Drawing for the job (mm, zero at the part's lowest x, y, z). Round coordinates to 2 decimals unless told otherwise and drop trailing zeros. Order: outer loops, then holes, each group sorted by start corner. A loop starts at its lowest first (then second) coordinate and runs counter-clockwise, first axis right, second up. Notation, with made-up numbers: (13, -13) -> (46, -13) arc R21 cw to (46, -9) -> close; hole circle Ø2 at (-18.5, 77). An arc over 180 degrees is marked (long way). Use CSV: the item, a comma, the result in double quotes.
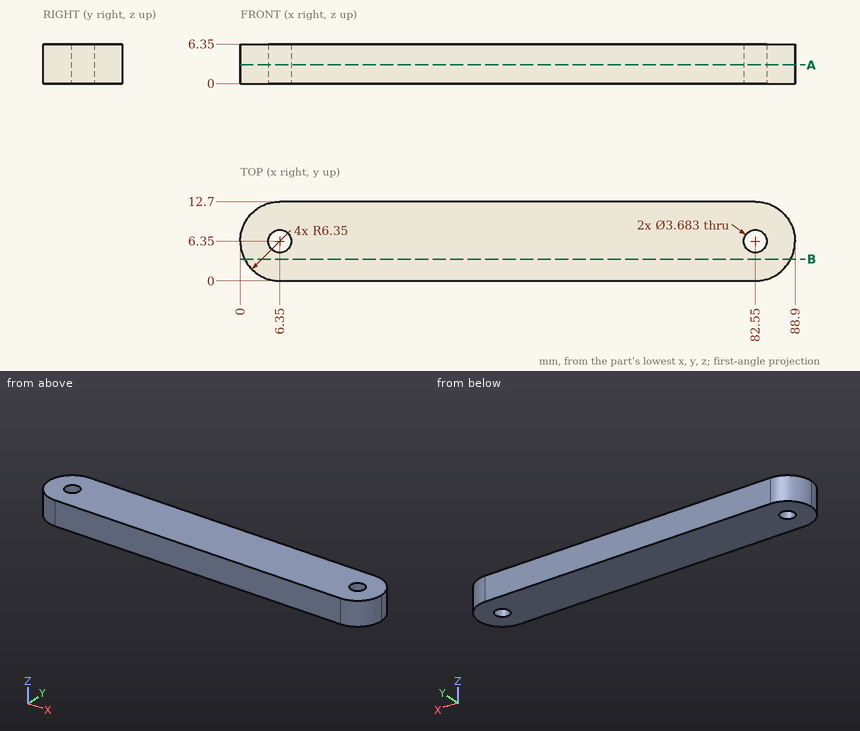
Q1. Cut at B-B (y = 3.5). Give the cut face in (x, z).
From the geometry:
outline,"(0.68, 0) -> (88.22, 0) -> (88.22, 6.35) -> (0.68, 6.35) -> close"
Q2. Probe line 1 along X through (y, z) = (6.35, 1.5); line 2 along X through (y, z) = (5.75, 1.5); line 3 along X through (y, z) = (8.5, 3) (3 decimals). List the from-to ranges inside material, lowest first.
From the geometry:
line 1,"x = 0 to 4.51, 8.19 to 80.71, 84.39 to 88.9"
line 2,"x = 0.03 to 4.61, 8.09 to 80.81, 84.29 to 88.87"
line 3,"x = 0.375 to 88.525"
Q3. Pin check, flat tips, straight feed: pin 1 (3.5 mm diameter, centred on x = 6.35, y = 6.35, fed in from -Z); pin 2 (1.5 mm diameter, centred on y = 3, z = 4, fed in from -X). Stop position of each tip, or through.
From the geometry:
pin 1,"passes through"
pin 2,"stops at x = 0.56"
Q4. Cut at A-A (z = 3). State how many separate pieces and enclosed holes the cut face has, plus the area to 3 significant figures.
From the geometry:
separate pieces,"1"
enclosed holes,"2"
area,"1,070 mm²"
